Verification items for this drawing (mm, ordinates from the low corner). A direction names the side the tool comes from. Round coordinates to 2 decimals unless told otherwise and drop trailing zeros. Loops run counter-clockwise (first coordinate to the right, second up) from the corner with the lowest first, then second, coordinate; pieces in that order, holes last. Notation, with made-up numbers: (-5.75, 42) - (53.25, 42) arc R15 cw to (53.25, 65) - close; hole circle Ø6 at (48, 51.5). An arc over 180 degrees is marked (long way). Put each result on its own line as item: value. Start each with the question number.
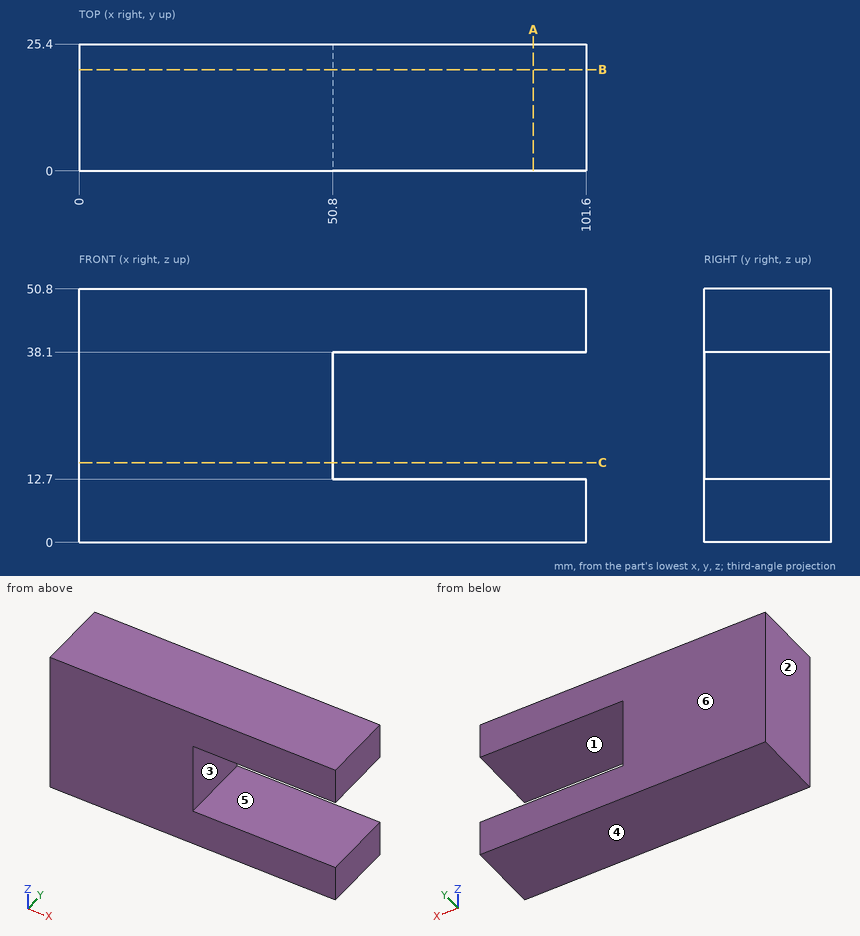
Q1. Set-up check for the marked faces 5 and 6: record each of +Z, -Z, +X, -X, +Y, -Y from which the full face is reachable in a straight line by a thin tool's end or side.
Q2. Cross-section at A-A on x = 91. Enter the section's corners in (y, z), and give its area (3 significant figures).
Q3. Depth check by flat-ended pin: pin 1 Ø7.5 at (y, z) = (15, 25) entering from +X. Enter the tip coordinate at first touch or a pass-through.
Q4. Cross-section at B-B on y = 20.25. Enter the section's corners in (x, z).
Q5. Material ranges on line 1 (Z direction, x = 92.5, y = 13.5); line 2 (X direction, y = 6.25, z = 30.5), recorded low to high. Write a range as from..to.
Q6. Cross-section at C-C on z = 16. Enter the section's corners in (x, y), and give its area (3 significant figures).
Q7. Draft check along Z on the marked faces 1, 2, 3 and 4. Enter one of: +Z half, -Z half, draft (parallel to the pull), parting line (faces both ways), or undercut.
Answer list:
1. face 5: +X, +Y, -Y
1. face 6: +Z, -Z, +X, -X, +Y
2. outline: (0, 0) - (25.4, 0) - (25.4, 12.7) - (0, 12.7) - close; (0, 38.1) - (25.4, 38.1) - (25.4, 50.8) - (0, 50.8) - close
2. area: 645 mm2
3. pin 1: stops at x = 50.8
4. outline: (0, 0) - (101.6, 0) - (101.6, 12.7) - (50.8, 12.7) - (50.8, 38.1) - (101.6, 38.1) - (101.6, 50.8) - (0, 50.8) - close
5. line 1: z = 0..12.7, 38.1..50.8
5. line 2: x = 0..50.8
6. outline: (0, 0) - (50.8, 0) - (50.8, 25.4) - (0, 25.4) - close
6. area: 1,290 mm2
7. face 1: undercut
7. face 2: draft
7. face 3: undercut
7. face 4: -Z half
